The listing builds one solid part. Answer for the finished solid, in the listing's coordinates (mm). A direction names the side the tool comes from. Give positions to 0.01 mm unless a question says otherwise; leave off trailing zeros. Loops run counter-clockwise (first coordinate to the right, second up) from the corner with the lowest first, then second, coordinate; pieces in that order, holes last. Notation, with made-up numbers: M 7,2 L 60,2 A30 cw 60,25 Z; hole C 35.5,7 d7. An arc over 180 degrees is marked long. Return JSON: item names as keys, results as strings.
from build123d import *

# Parameters (mm, degrees)
SKETCH1_R           = 21.082
BOSS_EXTRUDE1_DEPTH = 64.262
SKETCH2_W           = 42.164
SKETCH2_H           = 42.164
BOSS_EXTRUDE2_DEPTH = 49.657
BOSS_EXTRUDE3_DEPTH = 42.545


with BuildPart() as part:
    # Sketch1 → Boss-Extrude1 (new body)
    with BuildSketch(Plane(origin=(0, 0, 0), x_dir=(0, 0, -1), z_dir=(1, 0, 0))):
        Circle(SKETCH1_R)
    extrude(amount=BOSS_EXTRUDE1_DEPTH)

    # Sketch2 → Boss-Extrude2 (add)
    with BuildSketch(Plane(origin=(64.262, 0, 0), x_dir=(0, 0, -1), z_dir=(1, 0, 0))):
        Rectangle(SKETCH2_W, SKETCH2_H)
    extrude(amount=BOSS_EXTRUDE2_DEPTH)

    # Sketch3 → Boss-Extrude3 (add)
    with BuildSketch(Plane(origin=(113.919, 0, 0), x_dir=(0, 0, -1), z_dir=(1, 0, 0))):
        Polygon((7.332348419, 0), (3.666174209, 6.35), (-3.666174209, 6.35), (-7.332348419, 0), (-3.666174209, -6.35), (3.666174209, -6.35), align=None)
    extrude(amount=BOSS_EXTRUDE3_DEPTH)


solid = part.part
(1) The part is cut by section C-C (y = -8.5). Determine the outline of the cut face in (x, z).
Values follow:
{"outline": "M 0,-19.29 L 64.26,-19.29 L 64.26,-21.08 L 113.92,-21.08 L 113.92,21.08 L 64.26,21.08 L 64.26,19.29 L 0,19.29 Z"}
(2) Given pin 1 (8 mm diameter, centred on y = -9, z = 16.5, fed in from +X); pin 2 (3.5 mm diameter, centred on x = 130.5, z = 2, fed in from -Y); pin 3 (12 mm diameter, centred on x = 135.5, z = 9.5, fed in from +Y), each flat-ended and moving along its own axis, determine where each tip first touches the part or whether it passes through.
Values follow:
{"pin 1": "x = 113.92", "pin 2": "y = -6.35", "pin 3": "y = 6.35"}
(3) The part is cut by section B-B (z = 17.5). Determine the outline of the cut face in (x, y).
Values follow:
{"outline": "M 0,-11.76 L 64.26,-11.76 L 64.26,-21.08 L 113.92,-21.08 L 113.92,21.08 L 64.26,21.08 L 64.26,11.76 L 0,11.76 Z"}
(4) The part is cut by section A-A (y = 5). Determine the outline of the cut face in (x, z).
Values follow:
{"outline": "M 0,-20.48 L 64.26,-20.48 L 64.26,-21.08 L 113.92,-21.08 L 113.92,-4.45 L 156.46,-4.45 L 156.46,4.45 L 113.92,4.45 L 113.92,21.08 L 64.26,21.08 L 64.26,20.48 L 0,20.48 Z"}
(5) A tool of negligible diameter and unlimited length cuts with its end or side. For faces 1 (the flat face through (135, -6.35, 0)), 2 (the flat face through (134.894, 3.131, -5.525)), 3 (the cylindrical face through (31.68, 6.33, -20.11)), 4 (the flat face through (135, 6.35, 0)), 5 (the flat face through (64.262, -17, -17)), from which of +Z, -Z, +X, -X, +Y, -Y can it reach the whole face along a straight path? Write none if from no direction.
Values follow:
{"face 1": "+Z, -Z, +X, -Y", "face 2": "-Z, +X, +Y", "face 3": "-X", "face 4": "+Z, -Z, +X, +Y", "face 5": "-Z, -X, -Y"}
(6) Straight lines are drawn through the part: line 1 along X through (y, z) = (-15.5, 5); line 2 along Y through (x, z) = (120, 2.5); line 3 along Z through (x, y) = (33, -5.5). For each, find the intervals that lie inside material, in ascending order.
Values follow:
{"line 1": "0 to 113.92", "line 2": "-6.35 to 6.35", "line 3": "-20.35 to 20.35"}
